Autodesk Inventor part; units mm, degrees
ref_plane "YZ Plane" through (0, 0, 0) normal (1, 0, 0) x (0, 1, 0)
ref_plane "XZ Plane" through (0, 0, 0) normal (0, 1, 0) x (-1, 0, 0)
ref_plane "XY Plane" through (0, 0, 0) normal (0, 0, 1) x (1, 0, 0)
sketch "Sketch1" plane through (0, 0, 0) normal (0, 0, 1) x (1, 0, 0)
  arc A0 (-2.65, 0) -> (2.65, 0) centre (0, 0) ccw
  line L0 (-7.5, 9.35) -> (7.5, 9.35)
  line L1 (7.5, 9.35) -> (7.5, 4.85)
  line L2 (-7.5, 4.85) -> (-7.5, 9.35)
  line L3 (-2.65, 0) -> (-2.65, 0.85)
  line L4 (2.65, 0.85) -> (2.65, 0)
  line L5 (7.5, 4.85) -> (6.65, 4.85)
  line L6 (-6.65, 4.85) -> (-7.5, 4.85)
  line L7 (0, 0) -> (0, 9.35) construction
  arc A1 (-2.65, 0.85) -> (-6.65, 4.85) centre (-6.65, 0.85) ccw
  arc A2 (6.65, 4.85) -> (2.65, 0.85) centre (6.65, 0.85) ccw
  dimension "d0" = 2.65
  dimension "d1" = 4.5
  dimension "d2" = 15
  dimension "d3" = 12
  dimension "d4" = 4
extrude "Extrusion1" add sketch "Sketch1" along normal blind 9
shell "Shell1" thickness 1 removed faces 1 at (-2.5, 9.35, 3)
sketch "Sketch3" plane through (-7.5, 9.35, 0) normal (0, 1, 0) x (1, 0, 0)
  line L0 (1, -5.1) -> (1, -3.9)
  line L1 (14, -3.9) -> (14, -5.1)
  line L2 (11, -2.1) -> (4, -2.1)
  line L3 (4, -6.9) -> (11, -6.9)
  line L4 (11, -2.1) -> (4, -6.9) construction
  line L5 (4, -2.1) -> (11, -6.9) construction
  line L6 (14, -5.1) -> (11, -5.1)
  line L7 (4, -5.1) -> (1, -5.1)
  line L8 (1, -3.9) -> (4, -3.9)
  line L9 (11, -3.9) -> (14, -3.9)
  line L10 (4, -2.1) -> (4, -3.9)
  line L11 (4, -5.1) -> (4, -6.9)
  line L12 (11, -6.9) -> (11, -5.1)
  line L13 (11, -3.9) -> (11, -2.1)
  line L14 (14, -1) -> (14, -8)
  line L15 (1, -8) -> (1, -1)
  line L16 (14, -8) -> (1, -8)
  line L17 (7.5, -8) -> (7.5, -4.5) construction
  line L18 (1, -1) -> (14, -1)
  line L19 (7.5, -1) -> (7.5, -4.5) construction
  line L20 (4.8, -2.6486) -> (10.2, -2.6486)
  line L21 (10.2, -2.6486) -> (10.2, -6.3514)
  line L22 (10.2, -6.3514) -> (4.8, -6.3514)
  line L23 (4.8, -6.3514) -> (4.8, -2.6486)
  line L24 (4.8, -2.6486) -> (10.2, -6.3514) construction
  line L25 (10.2, -2.6486) -> (4.8, -6.3514) construction
  point P0 (7.5, 0)
  dimension "d8" = 1.2
  dimension "d9" = 7
  dimension "d10" = 4.8
  dimension "d11" = 0.8
extrude "Extrusion2" add sketch "Sketch3" against normal up to next contours L0 L8 L10 L2 L13 L9 L1 L6 L12 L3 L11 L7
properties part number "Boton de temperaturas" material "ABS Plastic"
The model under review builds one solid part; all positions refer to its coordinate system, in mm. A direction names the side the tool comes from. Round coordinates to 2 decimals unless told otherwise and drop trailing zeros. Write each loop counter-clockwise with the first axis right and the second up, starting at its lowest first coordinate (ties: lowest second). Pieces come first, ordered by that corner, then holes. Notation, with made-up numbers: M 37.25,-36 L 61.25,-36 A37 ccw 61.25,0 Z; hole C 11.5,-1 d9. An arc over 180 degrees is marked long. Use a Markdown table: item, result. Add a question column.
Q1. We need section C-C, the plane z = 3.25. State the section outline as (x, y) points, plus the area to 3 significant figures.
Q2. We need section D-D, the plane y = 6.25. State the section outline as (x, z) points, plus the area to 3 significant figures.
Q3. Machinability: for faces 4 (the face through (-0.1, 9.35, 2.4)), 5 (the face through (5, 8, 3.9)), 6 (the face through (2.65, 0.4, 4.4)), which of the approach directions +Z, -Z, +X, -X, +Y, -Y give a long, thin tool a straight path to every point of the face, cutting with its end or side? Answer none if there is none.
Q4. Insertion check: pin 1 (1 mm diameter, centred on x = 4, z = 1.5, fed in from -Y); pin 2 (0.7 mm diameter, centred on y = 0.5, z = 1.5, fed in from -X); pin 3 (4 mm diameter, centred on y = -0.5, z = 5.5, fed in from +X). Each pin has a flat end and moves straight along its axis. Give the tip position at first contact, or say it passes through.
Q5. To check wall thickness, follow line 1 (X direction, y = 7.5, z = 3); line 2 (X direction, y = 8.75, z = 6.75); line 3 (Z direction, x = -1.5, y = 1.25). State the ranges of each line that lie inside material, in increasing order.
Q6. We need section B-B, the plane x = 0. State the section outline as (y, z) points.
Q7. The part is to be moulded in two halves that separate along Z. For faces 1 (the face through (0, 5, 0)), 2 (the face through (-1.65, 0.4, 4.5)), 3 (the face through (0, 5, 9)), say which applies: pulls with the +Z half, pulls with the -Z half, needs draft (parallel to the pull), parting line crosses it, or undercut.
Q8. We need section A-A, the plane y = 0.5. State the section outline as (x, z) points, plus the area to 3 significant figures.
Findings below:
| question | item | result |
|---|---|---|
| 1 | outline | M -7.5,4.85 L -6.65,4.85 A4 cw -2.65,0.85 L -2.65,0 A2.65 ccw 2.65,0 L 2.65,0.85 A4 cw 6.65,4.85 L 7.5,4.85 L 7.5,9.35 L 6.5,9.35 L 6.5,5.85 A5 ccw 3.5,4.73 L 3.5,9.35 L 2.7,9.35 L 2.7,3.92 A5 ccw 1.65,0.85 L 1.65,0 A1.65 cw -1.65,0 L -1.65,0.85 A5 ccw -2.7,3.92 L -2.7,9.35 L -3.5,9.35 L -3.5,4.73 A5 ccw -6.5,5.85 L -6.5,9.35 L -7.5,9.35 Z |
| 1 | area | 39.3 mm² |
| 2 | outline | M -7.5,0 L 7.5,0 L 7.5,9 L -7.5,9 Z; hole M -6.5,1 L 6.5,1 L 6.5,3.9 L 3.5,3.9 L 3.5,2.1 L -3.5,2.1 L -3.5,3.9 L -6.5,3.9 Z; hole M -6.5,5.1 L -3.5,5.1 L -3.5,6.9 L 3.5,6.9 L 3.5,5.1 L 6.5,5.1 L 6.5,8 L -6.5,8 Z; hole M -2.7,2.65 L 2.7,2.65 L 2.7,6.35 L -2.7,6.35 Z |
| 2 | area | 64.8 mm² |
| 3 | face 4 | +Z, -Z, +X, -X, +Y |
| 3 | face 5 | +Y |
| 3 | face 6 | +Z, -Z, +X, -Y |
| 4 | pin 1 | stops at y = 3.32 |
| 4 | pin 2 | stops at x = -2.65 |
| 4 | pin 3 | stops at x = 2.7 |
| 5 | line 1 | x = -7.5 to -6.5, -3.5 to -2.7, 2.7 to 3.5, 6.5 to 7.5 |
| 5 | line 2 | x = -7.5 to -6.5, -3.5 to 3.5, 6.5 to 7.5 |
| 5 | line 3 | z = 0 to 1, 2.1 to 2.65, 6.35 to 6.9, 8 to 9 |
| 6 | outline | M -2.65,0 L 9.35,0 L 9.35,1 L -1.65,1 L -1.65,2.1 L 9.35,2.1 L 9.35,2.65 L -1.65,2.65 L -1.65,6.35 L 9.35,6.35 L 9.35,6.9 L -1.65,6.9 L -1.65,8 L 9.35,8 L 9.35,9 L -2.65,9 Z |
| 7 | face 1 | pulls with the -Z half |
| 7 | face 2 | undercut |
| 7 | face 3 | pulls with the +Z half |
| 8 | outline | M -2.65,0 L 2.65,0 L 2.65,9 L -2.65,9 Z; hole M -1.65,1 L 1.65,1 L 1.65,2.1 L -1.65,2.1 Z; hole M -1.65,2.65 L 1.65,2.65 L 1.65,6.35 L -1.65,6.35 Z; hole M -1.65,6.9 L 1.65,6.9 L 1.65,8 L -1.65,8 Z |
| 8 | area | 28.2 mm² |
